For this review, take the finished solid that the model builds, in its own axes (mm). Face numbers are marked on the shaded views. A direction names the side the tool comes from. Give positions to 0.01 mm unless a question says otherwise; leave off trailing zeros. Order: outer loops, then holes, each group sorted by start corner. A loop starts at its lowest first (then second) coordinate and runs counter-clockwise, first axis right, second up.
Item 1: Machinability: for the marked faces 1, 2, 3 and 4, which of the approach directions +Z, -Z, +X, -X, +Y, -Y give a long, thin tool a straight path to every point of the face, cutting with its end or side? Answer none if there is none.
Item 2: Consider section D-D (z = 14). Give the boundary of the cut face in (x, y).
Item 3: Consider section A-A (y = -5.5). Give the boundary of the cut face in (x, z).
Item 4: For probe 1 along Z at (x, y) = (-49.5, -49); probe 2 along X at (y, z) = (-6, 49); probe 3 along Z at (x, y) = (59, -41.5), list the stretches that pass through material, from the lowest coordinate up.
Item 5: Consider section C-C (z = 44). Give the boundary of the cut face in (x, y), plus the area to 3 significant figures.
Item 6: Consider section B-B (x = -32). Give the boundary of the cut face in (y, z).
Item 7: For P1, Ø2, axis at x = -63, z = 13.5, coming from the -Y side; P2, Ø8, axis at x = -24.5, y = -24.5, coming from the +Z side; P3, Ø5, axis at x = -49.5, y = -18.5, coming from the +Z side; P4, Ø12, axis at y = -45, z = 64.5, coming from the -X side, all flat-tipped, find the tip position at first contact; note any pin that passes through.
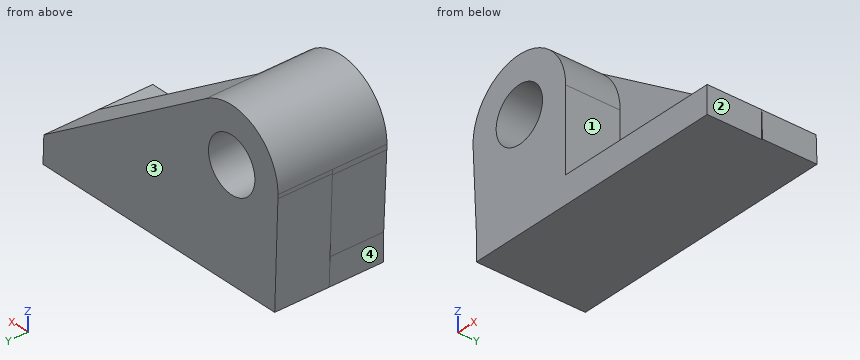
```python
from build123d import *

# Parameters (mm, degrees)
F1_DEPTH = 25.4
F2_R     = 12.7
F3_DEPTH = 25.4


with BuildPart() as f1:
    # F0 (on Front) → F1 (new body)
    with BuildSketch(Plane.XZ):
        with BuildLine():
            ThreePointArc((-24.391064, 71.906237), (-50.461929, 73.159197), (-63.872557, 50.7669))
            Line((-63.872557, 50.7669), (-63.806378, 48.934551))
            ThreePointArc((-63.806378, 48.934551), (-37.555786, 25.38345), (-13.072557, 50.7669))
            ThreePointArc((-13.072557, 50.7669), (-16.08026, 62.756272), (-24.391064, 71.906237))
        make_face()
        with BuildLine():
            ThreePointArc((-51.172557, 50.7669), (-38.472557, 63.4669), (-25.772557, 50.7669))
            ThreePointArc((-25.772557, 50.7669), (-38.472557, 38.0669), (-51.172557, 50.7669))
        make_face(mode=Mode.SUBTRACT)
        with BuildLine():
            Line((64.5026, 12.691725), (-24.391064, 71.906237))
            ThreePointArc((-24.391064, 71.906237), (-16.08026, 62.756272), (-13.072557, 50.7669))
            ThreePointArc((-13.072557, 50.7669), (-37.555786, 25.38345), (-63.806378, 48.934551))
            Line((-63.806378, 48.934551), (-62.039014, 0))
            Line((-62.039014, 0), (64.960986, 0))
            Line((64.960986, 0), (64.5026, 12.691725))
        make_face()
    extrude(amount=F1_DEPTH)

    # F2 (on face) → F3 (join)
    with BuildSketch(Plane.XZ.offset(25.4)):
        with BuildLine():
            Line((-13.072557, 12.691725), (-13.072557, 50.7669))
            ThreePointArc((-13.072557, 50.7669), (-16.08026, 62.756272), (-24.391064, 71.906237))
            ThreePointArc((-24.391064, 71.906237), (-50.461929, 73.159197), (-63.872557, 50.7669))
            Line((-63.872557, 50.7669), (-63.755025, 48.326241))
            Line((-63.755025, 48.326241), (-62.039014, 12.691725))
            Line((-62.039014, 12.691725), (-62.039014, 0))
            Line((-62.039014, 0), (64.5026, 0))
            Line((64.5026, 0), (64.5026, 12.691725))
            Line((64.5026, 12.691725), (-13.072557, 12.691725))
        make_face()
        with Locations((-38.472557, 50.7669)):
            Circle(F2_R, mode=Mode.SUBTRACT)
    extrude(amount=F3_DEPTH)


solid = f1.part
```
Resolved:
1. face 1: +Z, +X, -Y
1. face 2: +Z, -Z, +X, -Y
1. face 3: +Z, -Z, +X, -X, +Y
1. face 4: -Z, -X, -Y
2. outline: (-62.54, -25.4) - (-62.1, -25.4) - (-62.1, -50.8) - (-13.07, -50.8) - (-13.07, -25.4) - (62.54, -25.4) - (62.54, 0) - (-62.54, 0) - close
3. outline: (-63.87, 50.77) - (-63.81, 48.93) - (-62.04, 0) - (64.96, 0) - (64.5, 12.69) - (-24.39, 71.91) arc R25.4 ccw to start; hole circle Ø25.4 at (-38.47, 50.77)
4. probe 1: z = 0 to 44.47, 57.07 to 73.65
4. probe 2: x = -63.81 to -51.05, -25.9 to 10
4. probe 3: z = 0 to 12.69
5. outline: (-63.63, -25.4) - (-63.55, -25.4) - (-63.55, -50.8) - (-49.22, -50.8) - (-49.22, 0) - (-63.63, 0) - close; (-27.73, -50.8) - (-13.07, -50.8) - (-13.07, -25.4) - (17.5, -25.4) - (17.5, 0) - (-27.73, 0) - close
5. area: 2,250 mm2
6. outline: (-50.8, 0) - (0, 0) - (0, 39.84) - (-50.8, 39.84) - close; (-50.8, 61.69) - (0, 61.69) - (0, 75.33) - (-50.8, 75.33) - close
7. P1: stops at y = -50.8
7. P2: stops at z = 74.13
7. P3: stops at z = 74.69
7. P4: stops at x = -62.67
